```python
from build123d import *

# Parameters (mm, degrees)
SALIENTE_EXTRUIR1_DEPTH = 30


with BuildPart() as part:
    # Croquis1 → Saliente-Extruir1 (new body)
    with BuildSketch(Plane.XY):
        with BuildLine():
            Line((-145, -25), (145, -25))
            ThreePointArc((145, -25), (164.364916731, -17.912878475), (174.580398915, 0))
            ThreePointArc((174.580398915, 0), (164.364916731, 17.912878475), (145, 25))
            Line((145, 25), (-145, 25))
            ThreePointArc((-145, 25), (-164.364916731, 17.912878475), (-174.580398915, 0))
            ThreePointArc((-174.580398915, 0), (-164.364916731, -17.912878475), (-145, -25))
        make_face()
    extrude(amount=SALIENTE_EXTRUIR1_DEPTH)


solid = part.part
```
Input: part model. Units: mm. Frame: model coordinates. Give positions to 0.01 mm unless a question says otherwise; leave off trailing zeros. Order: outer loops, then holes, each group sorted by start corner. A loop starts at its lowest first (then second) coordinate and runs counter-clockwise, first axis right, second up. Notation, with made-up numbers: (89.25, 0.5) -> (130.25, 0.5) arc R28 ccw to (130.25, 30.5) -> close; hole circle Ø11 at (74, 82). An arc over 180 degrees is marked (long way). Write each question's results on one line, items separated by ' | '. Start each with the question number.
Item 1: Cut plane C-C on y = -20. Return the cut outline in (x, z), then the cut area to 4 significant figures.
Item 2: Cut plane B-B on y = 17. Return the cut outline in (x, z), then the cut area to 3 significant figures.
Item 3: Cut plane A-A on z = 21.25. Return the cut outline in (x, y).
Item 4: Contact query for flat-ended pins moving along their axis: P1, Ø1.5, axis at y = 13, z = 6.5, coming from the -X side; P2, Ø8, axis at y = -7, z = 20.5, coming from the -X side; P3, Ø1, axis at y = 16, z = 14, coming from the -X side. Output: stop coordinate, or through.
Item 5: Line query: line 1 (X direction, y = -3, z = 5.5); line 2 (X direction, y = -22, z = 5.75). Output: solid intervals per line, ascending.
Established:
1) outline: (-161.58, 0) -> (161.58, 0) -> (161.58, 30) -> (-161.58, 30) -> close | area: 9,695 mm^2
2) outline: (-165.4, 0) -> (165.4, 0) -> (165.4, 30) -> (-165.4, 30) -> close | area: 9,920 mm^2
3) outline: (-174.58, 0) arc R30 ccw to (-145, -25) -> (145, -25) arc R30 ccw to (174.58, 0) arc R30 ccw to (145, 25) -> (-145, 25) arc R30 ccw to start
4) P1: x = -169.54 | P2: x = -173.91 | P3: x = -166.9
5) line 1: -173.91 to 173.91 | line 2: -158.08 to 158.08
